```python
from build123d import *

# Parameters (mm, degrees)
SKETCH030_W      = 34.5
SKETCH030_H      = 19.2
PAD018_DEPTH     = 0.65
SKETCH031_W      = 31.32
SKETCH031_H      = 15.62
SKETCH031_W_2    = 29.42
SKETCH031_H_2    = 14.2
PAD019_DEPTH     = 0.05
SKETCH032_W      = 34.5
SKETCH032_H      = 23
PAD020_DEPTH     = 0.7
SKETCH033_W      = 33.5
SKETCH033_H      = 18.2
PAD021_DEPTH     = 0.25
PAD024_DEPTH     = 0.2
SKETCH038_W      = 12
SKETCH038_H      = 0.2
REVOLUTION_ANGLE = 180
SKETCH039_R      = 0.4
PAD025_DEPTH     = 0.2


with BuildPart() as part:
    # Sketch030 (on Face1 of CopyPad017) → Pad018 (new body)
    with BuildSketch(Plane(origin=(0, 0, 8.95), x_dir=(1, 0, 0), z_dir=(0, 0, -1))):
        with Locations((20.25, -28.15)):
            Rectangle(SKETCH030_W, SKETCH030_H)
    extrude(amount=PAD018_DEPTH)

    # Sketch031 (on Face5 of Pad018) → Pad019 (join)
    with BuildSketch(Plane.XY.offset(8.95)):
        with Locations((20.25, 28.01)):
            Rectangle(SKETCH031_W, SKETCH031_H)
        with Locations((20.25, 28.01)):
            Rectangle(SKETCH031_W_2, SKETCH031_H_2, mode=Mode.SUBTRACT)
    extrude(amount=PAD019_DEPTH)

    # Sketch032 (on Face5 of Pad019) → Pad020 (join)
    with BuildSketch(Plane(origin=(0, 0, 8.3), x_dir=(1, 0, 0), z_dir=(0, 0, -1))):
        with Locations((20.25, -30.05)):
            Rectangle(SKETCH032_W, SKETCH032_H)
    extrude(amount=PAD020_DEPTH)

    # Sketch033 (on Face13 of Pad020) → Pad021 (join)
    with BuildSketch(Plane(origin=(0, 0, 7.6), x_dir=(1, 0, 0), z_dir=(0, 0, -1))):
        with Locations((20.25, -28.15)):
            Rectangle(SKETCH033_W, SKETCH033_H)
    extrude(amount=PAD021_DEPTH)

    # Sketch037 (on Face13 of Pad021) → Pad024 (join)
    with BuildSketch(Plane(origin=(0, 0, 7.6), x_dir=(1, 0, 0), z_dir=(0, 0, -1))):
        Polygon((12.65, -37.25), (27.85, -37.25), (27.85, -41.05), (26.25, -41.05), (26.25, -43.61), (14.25, -43.61), (14.25, -41.05), (12.65, -41.05), align=None)
    extrude(amount=PAD024_DEPTH)

    # Sketch038 (on Face32 of Pad024) → Revolution (revolve)
    with BuildSketch(Plane(origin=(0, 43.61, 0), x_dir=(-1, 0, 0), z_dir=(0, 1, 0))):
        with Locations((-20.25, 7.5)):
            Rectangle(SKETCH038_W, SKETCH038_H)
    revolve(axis=Axis((26.262199, 43.61, 6.9), (-1, 0, 0)), revolution_arc=REVOLUTION_ANGLE)

    # Sketch039 (on Face27 of Revolution) → Pad025 (join)
    with BuildSketch(Plane.XY.offset(6.2)):
        Polygon((14.25, 43.61), (14.25, 43.406751), (9.25, 40.52), (9.25, 36.52), (31.25, 36.52), (31.25, 40.52), (26.25, 43.406751), (26.25, 43.61), align=None)
        with Locations((12.25, 41.27)):
            Circle(SKETCH039_R, mode=Mode.SUBTRACT)
        with Locations((28.25, 41.27)):
            Circle(SKETCH039_R, mode=Mode.SUBTRACT)
    extrude(amount=PAD025_DEPTH)


solid = part.part
```
Can you work these out from the model? Positions are in its coordinate system, mm. A direction names the side the tool comes from. Coordinates: 2 decimals unless noted, no trailing zeros. Loops run counter-clockwise (first coordinate to the right, second up) from the corner with the lowest first, then second, coordinate; pieces in that order, holes last. Notation, with made-up numbers: (81, 38.25) -> (97, 38.25) arc R26 ccw to (97, 70.25) -> close; hole circle Ø1 at (5.25, 40). An arc over 180 degrees is marked (long way). Answer as a JSON object with one key per item and string values.
1) Imagine slicing it at D-D (x = 28.25). Please give me the cut outline in (y, z), then the cut area to 3 significant figures.
Results:
{"outline": "(18.55, 7.6) -> (19.05, 7.6) -> (19.05, 7.35) -> (37.25, 7.35) -> (37.25, 7.6) -> (41.55, 7.6) -> (41.55, 8.3) -> (37.75, 8.3) -> (37.75, 8.95) -> (35.82, 8.95) -> (35.82, 9) -> (35.11, 9) -> (35.11, 8.95) -> (20.91, 8.95) -> (20.91, 9) -> (20.2, 9) -> (20.2, 8.95) -> (18.55, 8.95) -> close; (36.52, 6.2) -> (40.87, 6.2) -> (40.87, 6.4) -> (36.52, 6.4) -> close; (41.67, 6.2) -> (42.25, 6.2) -> (42.25, 6.4) -> (41.67, 6.4) -> close", "area": "34.2 mm^2"}
2) For faces 1 (the face through (20, 40, 7.4)), 2 (the face through (20, 40, 6.4)), 3 (the face through (20, 43, 7.6)), 4 (the face through (20, 18.55, 8)), 5 (the face through (12.5, 37.7, 7.6)), which set-ups out of +Z, -Z, +X, -X, +Y, -Y let a thin tool reach every point of the face, with its end or its side?
Results:
{"face 1": "+X, -X", "face 2": "+X, -X, -Y", "face 3": "+Z, +X, -X, +Y", "face 4": "+Z, -Z, +X, -X, -Y", "face 5": "none"}
3) Imagine slicing it at B-B (y = 42.75). Please give me the cut outline in (x, z), then the cut area to 4 significant figures.
Results:
{"outline": "(13.11, 6.2) -> (27.39, 6.2) -> (27.39, 6.4) -> (13.11, 6.4) -> close; (14.25, 7.4) -> (26.25, 7.4) -> (26.25, 7.6) -> (14.25, 7.6) -> close", "area": "5.255 mm^2"}
4) If I drill on line 1 (Z direction, x = 21, y = 40.75); line 2 (X direction, y = 41.27, z = 6.35); line 3 (Y direction, x = 5, z = 8), over which ranges is the centre line in solid material (lowest first)?
Results:
{"line 1": "z = 6.2 to 6.4, 7.4 to 8.3", "line 2": "x = 10.55 to 11.85, 12.65 to 27.85, 28.65 to 29.95", "line 3": "y = 18.55 to 41.55"}
5) Thinking about a two-plate mould opening in Z: for faces 6 (the face through (20, 40, 6.2)), 7 (the face through (20, 28, 8.95)), 8 (the face through (20.17, 44.11, 6.91)), 9 (the face through (3, 30, 8)), which applies, pulls with the +Z half, pulls with the -Z half, needs draft (parallel to the pull), parting line crosses it, or undercut?
Results:
{"face 6": "pulls with the -Z half", "face 7": "pulls with the +Z half", "face 8": "undercut", "face 9": "needs draft"}
6) Imagine slicing it at C-C (y = 33). Please give me the cut outline in (x, z).
Results:
{"outline": "(3, 7.6) -> (3.5, 7.6) -> (3.5, 7.35) -> (37, 7.35) -> (37, 7.6) -> (37.5, 7.6) -> (37.5, 8.95) -> (35.91, 8.95) -> (35.91, 9) -> (34.96, 9) -> (34.96, 8.95) -> (5.54, 8.95) -> (5.54, 9) -> (4.59, 9) -> (4.59, 8.95) -> (3, 8.95) -> close"}
7) For P1, Ø11.5, axis at x = 26, y = 25.5, coming from the -Z side; P2, Ø6, axis at x = 20.5, y = 31, coming from the +Z side; P3, Ø1.9, axis at x = 17, y = 39, coming from the +Z side, each with a flat end and sliding along its axis, tell me the tip position at first contact or that it passes through.
Results:
{"P1": "stops at z = 7.35", "P2": "stops at z = 8.95", "P3": "stops at z = 8.3"}
8) Imagine slicing it at A-A (x = 11.5). Please give me the cut outline in (y, z).
Results:
{"outline": "(18.55, 7.6) -> (19.05, 7.6) -> (19.05, 7.35) -> (37.25, 7.35) -> (37.25, 7.6) -> (41.55, 7.6) -> (41.55, 8.3) -> (37.75, 8.3) -> (37.75, 8.95) -> (35.82, 8.95) -> (35.82, 9) -> (35.11, 9) -> (35.11, 8.95) -> (20.91, 8.95) -> (20.91, 9) -> (20.2, 9) -> (20.2, 8.95) -> (18.55, 8.95) -> close; (36.52, 6.2) -> (41.82, 6.2) -> (41.82, 6.4) -> (36.52, 6.4) -> close"}
